Verification items for the finished model (mm, model axes). A direction names the side the tool comes from. Coordinates: 2 decimals unless noted, no trailing zeros. Order: outer loops, then holes, each group sorted by start corner. A loop starts at its lowest first (then second) coordinate and runs counter-clockwise, first axis right, second up. Notation, with made-up numbers: M 32,67.25 L 59,67.25 A28 cw 59,102.25 Z; hole C 5,14.25 d7. An arc over 180 degrees is marked long. Return JSON: item names as keys, results as strings.
```python
from build123d import *

# Parameters (mm, degrees)
ESQUISSE1_R                  = 26.5
EXTRUSION1_DEPTH             = 1
ENL_V_MAT_EXTRU_1_DEPTH      = 2
R_P_TITION_CIRCULAIRE1_COUNT = 13
ESQUISSE3_R                  = 21
EXTRUSION2_DEPTH             = 2.125
ESQUISSE4_R                  = 16
ENL_V_MAT_EXTRU_2_DEPTH      = 3.125
ENL_V_MAT_EXTRU_2_DEPTH_BACK = 3.125
CHANFREIN1_SIZE              = 0.5


with BuildPart() as part:
    # Esquisse1 → Extrusion1 (new body, symmetric)
    with BuildSketch(Plane.XY):
        Circle(ESQUISSE1_R)
    extrude(amount=EXTRUSION1_DEPTH, both=True)

    # Esquisse2 → Enlèv. mat.-Extru.1 (cut, symmetric)
    with BuildSketch(Plane.XY):
        with BuildLine():
            Line((-5.219783613, 25.98083638), (-3.276608177, 23.205694255))
            ThreePointArc((-3.276608177, 23.205694255), (0.898959157, 21.60232474), (3.95048165, 24.87254902))
            Line((3.95048165, 24.87254902), (4.156862745, 26.171940931))
            ThreePointArc((4.156862745, 26.171940931), (-0.53998188, 26.494497911), (-5.219783613, 25.98083638))
        make_face()
    enl_v_mat_extru_1 = extrude(amount=ENL_V_MAT_EXTRU_1_DEPTH, both=True, mode=Mode.SUBTRACT)

    # Répétition circulaire1: Enlèv. mat.-Extru.1 ×13 about axis
    r_p_tition_circulaire1_axis = Axis((0, 0, 0), (0, 0, 1))
    for i in range(1, R_P_TITION_CIRCULAIRE1_COUNT):
        add(enl_v_mat_extru_1.rotate(r_p_tition_circulaire1_axis, i * 360 / R_P_TITION_CIRCULAIRE1_COUNT), mode=Mode.SUBTRACT)

    # Esquisse3 → Extrusion2 (add, symmetric)
    with BuildSketch(Plane.XY):
        Circle(ESQUISSE3_R)
    extrude(amount=EXTRUSION2_DEPTH, both=True)

    # Esquisse4 → Enlèv. mat.-Extru.2 (cut, two sides)
    with BuildSketch(Plane.XY) as enl_v_mat_extru_2_sk:
        Circle(ESQUISSE4_R)
    extrude(amount=ENL_V_MAT_EXTRU_2_DEPTH, mode=Mode.SUBTRACT)
    extrude(enl_v_mat_extru_2_sk.sketch, amount=-ENL_V_MAT_EXTRU_2_DEPTH_BACK, mode=Mode.SUBTRACT)

    # Chanfrein1
    chanfrein1_edges = [part.edges().sort_by_distance(p)[0] for p in [
        (-21, 0, -2.125),
        (-21, 0, 2.125),
        (-16, 0, -2.125),
        (-16, 0, 2.125),
    ]]
    chamfer(chanfrein1_edges, length=CHANFREIN1_SIZE)


solid = part.part
```
Q1. Tool access check on faces 1 (the face through (19.511, -15.597, 0.014)), 2 (the face through (-21.5, -12.71, 0.01)), 3 (the face through (-15.21, 19.81, 0.01)). Record the directions out of +Z, -Z, +X, -X, +Y, -Y that give a thin tool (end or side, any length) a straight path to the whole face; none if there is none.
Values:
{"face 1": "+Z, -Z, -Y", "face 2": "+Z, -Z, -X", "face 3": "+Z, -Z, +Y"}
Q2. Draft check along X on faces 4 (the face through (1, 17, -2.125)), 5 (the face through (-6.84, 25.6, 0.01)), 6 (the face through (0.834, 21.588, 0.014)), 7 (the face through (24.59, 9.88, 0.01)). Enter one of: pulls with the +X half, pulls with the -X half, needs draft (parallel to the pull), parting line crosses it, or undercut.
Values:
{"face 4": "needs draft", "face 5": "pulls with the -X half", "face 6": "undercut", "face 7": "pulls with the +X half"}
Q3. Material ranges on line 1 along Y through (x, z) = (0, 0.8); line 2 along X through (y, z) = (20, 0.4); line 3 along Z through (x, y) = (16, -14.5), recorded low to high.
Values:
{"line 1": "-26.5 to -16, 16 to 21.5", "line 2": "-17.39 to -15.57, -8.79 to 8.79, 14.91 to 17.39", "line 3": "-1 to 1"}
Q4. Cross-section at A-A, the plane x = 0. Record the boundary of the cut face in (y, z) (3 decimals), and give its area (3 significant figures).
Values:
{"outline": "M -26.5,-1 L -21,-1 L -21,-1.625 L -20.5,-2.125 L -16.5,-2.125 L -16,-1.625 L -16,1.625 L -16.5,2.125 L -20.5,2.125 L -21,1.625 L -21,1 L -26.5,1 Z; M 16,-1.625 L 16.5,-2.125 L 20.5,-2.125 L 21,-1.625 L 21,-1 L 21.5,-1 L 21.5,1 L 21,1 L 21,1.625 L 20.5,2.125 L 16.5,2.125 L 16,1.625 Z", "area": "53.5 mm^2"}
Q5. Go/stop test with a flat-tipped pin: pin 1 (1.5 mm diameter, centred on x = 11, y = -18.5, fed in from +Z). Record where the tip stops, or that it passes through.
Values:
{"pin 1": "z = 1.85"}
